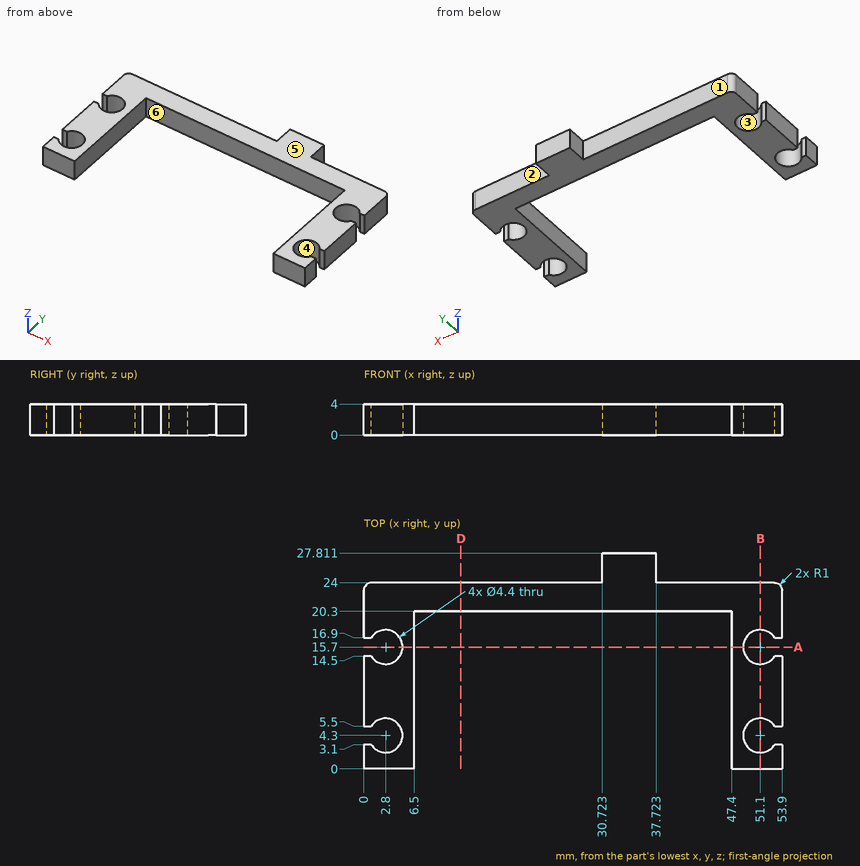
Verification items for this drawing (mm, ordinates from the low corner). A direction names the side the tool comes from. Coordinates: 2 decimals unless noted, no trailing zeros. Loops run counter-clockwise (first coordinate to the right, second up) from the corner with the lowest first, then second, coordinate; pieces in that order, holes last.
Item 1: Sectioned sample at B-B, the plane x = 51.1. Record the boundary of the cut face in (y, z).
Item 2: Thickness scan on line 1 (Y direction, x = 51.1, z = 1.9); line 2 (X direction, y = 15.7, z = 2); line 3 (Y direction, x = 4.5, z = 2.4) (1 decimal). Record the ranges inside material, lowest first.
Item 3: Access from +Z, -Z, +X, -X, +Y, -Y to the whole of each face (thin tool, end or side, straight path). Record for the marked faces 1, 2 and 3.
Item 4: Go/stop test with flat-tipped pins: pin 1 Ø1.1 at (x, z) = (53.5, 2) entering from +Y; pin 2 Ø1.9 at (y, z) = (25.5, 2) entering from -X; pin 3 Ø1.9 at (y, z) = (25.5, 1.5) entering from +X. Record where each tip stops, or that it passes through.
Item 5: Release check for a two-part mould opening along Y. For the marked faces 4, 5 and 6 record: released by +Y, released by -Y, zero draft, split by the parting line, or undercut.
Item 6: Sectioned sample at D-D, the plane x = 12.5. Record the boundary of the cut face in (y, z).
Item 7: Sectioned sample at A-A, the plane y = 15.7. Record the boundary of the cut face in (x, z).
Check result:
1. outline: (0, 0) - (2.1, 0) - (2.1, 4) - (0, 4) - close; (6.5, 0) - (13.5, 0) - (13.5, 4) - (6.5, 4) - close; (17.9, 0) - (24, 0) - (24, 4) - (17.9, 4) - close
2. line 1: y = 0 to 2.1, 6.5 to 13.5, 17.9 to 24
2. line 2: x = 5 to 6.5, 47.4 to 48.9
2. line 3: y = 0 to 2.9, 5.7 to 14.3, 17.1 to 24
3. face 1: +Z, -Z, -X, +Y
3. face 2: +Z, -Z, +X, +Y
3. face 3: +Z, -Z
4. pin 1: stops at y = 24
4. pin 2: stops at x = 30.72
4. pin 3: stops at x = 37.72
5. face 4: undercut
5. face 5: zero draft
5. face 6: released by -Y
6. outline: (20.3, 0) - (24, 0) - (24, 4) - (20.3, 4) - close
7. outline: (5, 0) - (6.5, 0) - (6.5, 4) - (5, 4) - close; (47.4, 0) - (48.9, 0) - (48.9, 4) - (47.4, 4) - close
